Model file for the job. Use its own axes, mm. A direction names the side the tool comes from. Coordinates: 2 decimals unless noted, no trailing zeros. Order: outer loops, then holes, each group sorted by start corner. A loop starts at its lowest first (then second) coordinate and runs counter-clockwise, first axis right, second up. Notation, with made-up numbers: (8.5, -16.75) -> (31.5, -16.75) arc R22 ccw to (31.5, 16.25) -> close; hole circle Ø7 at (81.5, 23). An arc over 180 degrees is marked (long way). Return JSON: item names as keys, results as strings. Group by question number.
1) Which spindle directions (+Z, -Z, +X, -X, +Y, -Y) get a long thin tool onto all of the face, cutting with end or side? Do faces 4 (the flat face through (71, -13, 0.209)), 5 (the flat face through (-8, -13, 0.209)), 6 (the flat face through (19.05, -13, 25)), 7 (the flat face through (57, -13, 12.909)). Say none if no direction does.
2) Cut at B-B (z = 5.5). Write the cut outline in (x, y).
3) Cut at C-C (x = 58). Write the cut outline in (y, z), and give its area (3 significant figures).
4) Pull direction Z, two halves, no side cores. Call faces 1 (the cylindrical face through (76.197, -12.979, 6.648)), 2 (the cylindrical face through (31.928, -12.421, 44.656)), 3 (the cylindrical face through (31.928, -9.77, 26.326)): +Z half, -Z half, draft (parallel to the pull), parting line (faces both ways), or undercut.
5) Cut at A-A (y = -12.7). Write the cut outline in (x, z).
6) Probe line 1 (X direction, y = -12.7, z = 7); line 2 (Y direction, x = 63.5, z = 9.5); line 3 (Z direction, x = 28, y = -12.7). List the from-to ranges inside material, lowest first.
7) Flat gauge pins, fed straight in: pin 1 (10 mm diameter, centred on x = -4.5, y = -13.5, fed in from -Z); pin 2 (7.5 mm diameter, centred on x = 5.5, y = -14.5, fed in from +Z); pin 3 (6 mm diameter, centred on x = 17.5, y = -16, fed in from +Z). Where does each tip first touch, or does it go through?
8) Cut at D-D (z = 16). Write the cut outline in (x, y), and give its area (3 significant figures).
from build123d import *

# Parameters (mm, degrees)
F0_W      = 63.5
F0_H      = 38.1
F1_DEPTH  = 25.4
F3_DEPTH  = 25.4
F5_DEPTH  = 25.4
F7_DEPTH  = 12.7
F9_DEPTH  = 12.7
F10_R     = 6.35
F11_DEPTH = 25.4
F12_R     = 6.35
F13_DEPTH = 25.4
F14_R     = 6.35
F15_DEPTH = 25.4


with BuildPart() as f1:
    # F0 (on Front) → F1 (new body)
    with BuildSketch(Plane.XZ):
        with Locations((31.75, 19.05)):
            Rectangle(F0_W, F0_H)
    extrude(amount=F1_DEPTH)

    # F2 (on face) → F3 (cut)
    with BuildSketch(Plane.XZ.offset(25.4)):
        Polygon((0, 38.1), (0, 12.909415), (19.05, 12.909415), (19.05, 31.959415), (44.45, 31.959415), (44.45, 12.909415), (63.5, 12.909415), (63.5, 38.1), align=None)
    extrude(amount=-F3_DEPTH, mode=Mode.SUBTRACT)

    # F4 (on face) → F5 (join)
    with BuildSketch(Plane.YZ.offset(44.45)):
        with BuildLine():
            Line((-25.4, 31.959415), (0, 31.959415))
            ThreePointArc((0, 31.959415), (-12.7, 44.659415), (-25.4, 31.959415))
        make_face()
    extrude(amount=-F5_DEPTH)

    # F6 (on face) → F7 (join)
    with BuildSketch(Plane.XY.offset(12.909415)):
        with BuildLine():
            Line((0, -25.4), (0, 0))
            ThreePointArc((0, 0), (-12.7, -12.7), (0, -25.4))
        make_face()
    extrude(amount=-F7_DEPTH)

    # F8 (on face) → F9 (join)
    with BuildSketch(Plane.XY.offset(12.909415)):
        with BuildLine():
            Line((63.5, 0), (63.5, -25.4))
            ThreePointArc((63.5, -25.4), (76.2, -12.7), (63.5, 0))
        make_face()
    extrude(amount=-F9_DEPTH)

    # F10 (on face) → F11 (cut)
    with BuildSketch(Plane.YZ.offset(44.45)):
        with Locations((-12.7, 31.959415)):
            Circle(F10_R)
    extrude(amount=-F11_DEPTH, mode=Mode.SUBTRACT)

    # F12 (on face) → F13 (cut)
    with BuildSketch(Plane.XY.offset(12.909415)):
        with Locations((63.5, -12.7)):
            Circle(F12_R)
    extrude(amount=-F13_DEPTH, mode=Mode.SUBTRACT)

    # F14 (on face) → F15 (cut)
    with BuildSketch(Plane.XY.offset(12.909415)):
        with Locations((0, -12.7)):
            Circle(F14_R)
    extrude(amount=-F15_DEPTH, mode=Mode.SUBTRACT)


solid = f1.part
Answers below:
{
 "1": {"face 4": "-Z, +X, +Y, -Y", "face 5": "-Z, -X, +Y, -Y", "face 6": "+Z, -X, +Y, -Y", "face 7": "+Z, +X, +Y, -Y"},
 "2": {"outline": "(0, -25.4) -> (63.5, -25.4) arc R12.7 ccw to (63.5, 0) -> (0, 0) arc R12.7 ccw to start; hole circle Ø12.7 at (0, -12.7); hole circle Ø12.7 at (63.5, -12.7)"},
 "3": {"outline": "(-25.4, 0) -> (-15.87, 0) -> (-15.87, 12.91) -> (-25.4, 12.91) -> close; (-9.53, 0) -> (0, 0) -> (0, 12.91) -> (-9.53, 12.91) -> close", "area": "246 mm^2"},
 "4": {"face 1": "draft", "face 2": "+Z half", "face 3": "undercut"},
 "5": {"outline": "(-12.7, 0.21) -> (-6.35, 0.21) -> (-6.35, 12.91) -> (-12.7, 12.91) -> close; (6.35, 0) -> (57.15, 0) -> (57.15, 12.91) -> (44.45, 12.91) -> (44.45, 25.61) -> (19.05, 25.61) -> (19.05, 12.91) -> (6.35, 12.91) -> close; (19.05, 38.31) -> (44.45, 38.31) -> (44.45, 44.66) -> (19.05, 44.66) -> close; (69.85, 0.21) -> (76.2, 0.21) -> (76.2, 12.91) -> (69.85, 12.91) -> close"},
 "6": {"line 1": "x = -12.7 to -6.35, 6.35 to 57.15, 69.85 to 76.2", "line 2": "y = -25.4 to -19.05, -6.35 to 0", "line 3": "z = 0 to 25.61, 38.31 to 44.66"},
 "7": {"pin 1": "stops at z = 0.21", "pin 2": "stops at z = 12.91", "pin 3": "stops at z = 44.64"},
 "8": {"outline": "(19.05, -25.4) -> (44.45, -25.4) -> (44.45, 0) -> (19.05, 0) -> close", "area": "645 mm^2"}
}
